from build123d import *

# Parameters (mm, degrees)
SZKIC1_R                    = 81
DODANIE_WYCI_GNI_CIE1_DEPTH = 50
SKORUPA1_T                  = -6
WYTNIJ_WYCI_GNI_CIE1_DEPTH  = 8
SZYK_KO_OWY1_COUNT          = 8
SZKIC5_R                    = 30
SZKIC5_R_2                  = 5.25
WYTNIJ_WYCI_GNI_CIE2_DEPTH  = 6
SZKIC6_R                    = 1.5
WYTNIJ_WYCI_GNI_CIE3_DEPTH  = 10
SZYK_KO_OWY2_COUNT          = 8
SFAZOWANIE1_SIZE            = 15
SFAZOWANIE1_SIZE2           = 8.660254038
SFAZOWANIE2_SIZE            = 15
SFAZOWANIE2_SIZE2           = 8.660254038


with BuildPart() as part:
    # Szkic1 → Dodanie-wyciągnięcie1 (new body)
    with BuildSketch(Plane.XY):
        Circle(SZKIC1_R)
    extrude(amount=DODANIE_WYCI_GNI_CIE1_DEPTH)

    # Skorupa1
    skorupa1_openings = [part.faces().sort_by_distance(p)[0] for p in [
        (0, 0, 0),
    ]]
    offset(amount=SKORUPA1_T, openings=skorupa1_openings, kind=Kind.INTERSECTION)

    # Szkic2 → Wytnij-wyciągnięcie1 (cut)
    with BuildSketch(Plane(origin=(0, 0, 0), x_dir=(-1, 0, 0), z_dir=(0, 0, -1))):
        with BuildLine():
            Line((5, 69.821200219), (5, 85.854528128))
            ThreePointArc((5, 85.854528128), (0, 86), (-5, 85.854528128))
            Line((-5, 85.854528128), (-5, 69.821200219))
            ThreePointArc((-5, 69.821200219), (0, 70), (5, 69.821200219))
        make_face()
    wytnij_wyci_gni_cie1 = extrude(amount=-WYTNIJ_WYCI_GNI_CIE1_DEPTH, mode=Mode.SUBTRACT)

    # Szyk kołowy1: Wytnij-wyciągnięcie1 ×8 about axis
    szyk_ko_owy1_axis = Axis((0, 0, 0), (0, 0, 1))
    for i in range(1, SZYK_KO_OWY1_COUNT):
        add(wytnij_wyci_gni_cie1.rotate(szyk_ko_owy1_axis, i * 360 / SZYK_KO_OWY1_COUNT), mode=Mode.SUBTRACT)

    # Szkic5 → Wytnij-wyciągnięcie2 (cut)
    with BuildSketch(Plane.XY.offset(50)):
        Circle(SZKIC5_R)
        with Locations((0, 50)):
            Circle(SZKIC5_R_2)
        with Locations((50, 0)):
            Circle(SZKIC5_R_2)
        with Locations((0, -50)):
            Circle(SZKIC5_R_2)
        with Locations((-50, 0)):
            Circle(SZKIC5_R_2)
    extrude(amount=-WYTNIJ_WYCI_GNI_CIE2_DEPTH, mode=Mode.SUBTRACT)

    # Szkic6 → Wytnij-wyciągnięcie3 (cut)
    with BuildSketch(Plane(origin=(0, 0, 0), x_dir=(-1, 0, 0), z_dir=(0, 0, -1))):
        with Locations((-29.849307724, 72.062603536)):
            Circle(SZKIC6_R)
    wytnij_wyci_gni_cie3 = extrude(amount=-WYTNIJ_WYCI_GNI_CIE3_DEPTH, mode=Mode.SUBTRACT)

    # Szyk kołowy2: Wytnij-wyciągnięcie3 ×8 about axis
    szyk_ko_owy2_axis = Axis((0, 0, 0), (0, 0, 1))
    for i in range(1, SZYK_KO_OWY2_COUNT):
        add(wytnij_wyci_gni_cie3.rotate(szyk_ko_owy2_axis, i * 360 / SZYK_KO_OWY2_COUNT), mode=Mode.SUBTRACT)

    # Sfazowanie1
    sfazowanie1_edges = [part.edges().sort_by_distance(p)[0] for p in [
        (-75, 0, 44),
    ]]
    sfazowanie1_side = [part.faces().sort_by_distance(p)[0] for p in [
        (-75, 0, 22),
    ]]
    chamfer(sfazowanie1_edges, length=SFAZOWANIE1_SIZE, length2=SFAZOWANIE1_SIZE2, reference=sfazowanie1_side[0])

    # Sfazowanie2
    sfazowanie2_edges = [part.edges().sort_by_distance(p)[0] for p in [
        (-81, 0, 50),
    ]]
    sfazowanie2_side = [part.faces().sort_by_distance(p)[0] for p in [
        (-81, 0, 25),
    ]]
    chamfer(sfazowanie2_edges, length=SFAZOWANIE2_SIZE, length2=SFAZOWANIE2_SIZE2, reference=sfazowanie2_side[0])


solid = part.part
Design review of the part built by this model. Coordinates are the model's own, in mm. A direction names the side the tool comes from. Give positions to 0.01 mm unless a question says otherwise; leave off trailing zeros. Loops run counter-clockwise (first coordinate to the right, second up) from the corner with the lowest first, then second, coordinate; pieces in that order, holes last. Notation, with made-up numbers: M 34,47.25 L 68,47.25 A32 cw 68,83.25 Z; hole C 76,-23.5 d9. An arc over 180 degrees is marked long. One line per question, with ' | ' between items. Start each with the question number.
1. To check wall thickness, follow L1, parallel to Y at x = 51, z = 39; L2, parallel to X at y = 39, z = 8.5; L3, parallel to Y at x = -25.5, z = 27. State the ranges of each line that lie inside material, in increasing order.
2. Insertion check: P1, Ø1, axis at x = 62, y = -33, coming from the -Z side; P2, Ø1.9, axis at x = -79.5, y = -1, coming from the -Z side; P3, Ø1.5, axis at x = 37, z = 12.5, coming from the +Y side. Each pin has a flat end and moves straight along its axis. Give the tip position at first contact, or say it passes through.
3. The part is to be moulded in two halves that separate along Y. For faces 1 (the face through (-58.606, -51.535, 3.944)), 2 (the face through (-78, -5, 4)), 3 (the face through (-29, 70, 0)), 4 (the face through (30.806, 59.228, 43.272)), say which applies: released by +Y, released by -Y, zero draft, split by the parting line, or undercut.
4. Add section C-C (z = 15.5). Write out the cut boundary in (x, y).
5. Add section A-A (x = 0). Write out the cut boundary in (y, z), plus the area to 3 significant figures.
6. For faces 5 (the face through (58.55, -51.48, 3.94)), 6 (the face through (55, -55, 8)), 7 (the face through (78, 0, 8)), 8 (the face through (0, 78, 8)), 9 (the face through (-71, 28, 0)), list the 3-axis set-ups (+Z, -Z, +X, -X, +Y, -Y) from which the entire face can be reached by the end or side of a thin tool; tool diameter is ignored.
Worked out:
1) L1: y = -59.93 to -46.81, 46.81 to 59.93 | L2: x = -70.99 to -64.06, 64.06 to 70.99 | L3: y = -76.88 to -70.53, 70.53 to 76.88
2) P1: stops at z = 36.39 | P2: stops at z = 8 | P3: stops at y = 72.44
3) face 1: released by -Y | face 2: undercut | face 3: zero draft | face 4: undercut
4) outline: C 0,0 d162; hole C 0,0 d150
5) outline: M -81,8 L -75,8 L -75,29 L -66.34,44 L -55.25,44 L -55.25,50 L -72.34,50 L -81,35 Z; M -44.75,44 L -30,44 L -30,50 L -44.75,50 Z; M 30,44 L 44.75,44 L 44.75,50 L 30,50 Z; M 55.25,44 L 66.34,44 L 75,29 L 75,8 L 81,8 L 81,35 L 72.34,50 L 55.25,50 Z | area: 918 mm²
6) face 5: -Z, -Y | face 6: -Z | face 7: -Z, +X, -X | face 8: -Z, +Y, -Y | face 9: -Z, +X, -X, +Y, -Y
